Model file for the job. Use its own axes, mm. A direction names the side the tool comes from. Give positions to 0.01 mm unless a question says otherwise; leave off trailing zeros. Order: outer loops, then holes, each group sorted by start corner. A loop starts at its lowest first (then second) coordinate and runs counter-clockwise, first axis right, second up. Notation, with made-up numbers: M 45.5,-1.75 L 63.5,-1.75 A14 ccw 63.5,11.25 Z; hole C 46.25,-16.75 d2. An arc over 180 degrees is marked long. Return JSON: item names as keys, results as strings. Group by question number.
1. Slice it at A-A on y = 2. List the corners of the cut face in (x, z), then the cut area to 3 significant figures.
2. Two-plate mould, pull along X, no slides. Class faces 1 (the face through (-11.4, -20.43, -1.23)), 2 (the face through (-10, 23, 1)), 3 (the face through (11, -1.1, -2)), 4 (the face through (11.43, 24.4, -1.27)): released by +X, released by -X, zero draft, split by the parting line, or undercut.
3. Slice it at C-C on z = -1.6. List the corners of the cut face in (x, y), then the cut area to 3 significant figures.
4. Slice it at D-D on y = -16. List the corners of the cut face in (x, z), then the cut area to 3 significant figures.
5. Wall check: probe 1 along Y at (x, z) = (2.75, 0.35); probe 2 along X at (y, z) = (-15, 0.1); probe 3 along Z at (x, y) = (1.75, 18). Give the ranges that are in metal, low to high. Write a range as [from, to].
6. Slice it at B-B on x = 1.75. List the corners of the cut face in (y, z), then the cut area to 4 significant figures.
7. Pin check, flat tips, straight feed: pin 1 (0.6 mm diameter, centred on x = 11.5, z = -1.5, fed in from +Y); pin 2 (3 mm diameter, centred on y = 3, z = -1.5, fed in from +X); pin 3 (1.3 mm diameter, centred on y = 3.5, z = -2, fed in from -X); pin 4 (1 mm diameter, centred on x = 11, z = -2, fed in from -Y). Stop position of each tip, or through.
8. 3-axis set-ups, long thin cutter, end or side, ignore diameter. For faces 5 (the face through (11.4, -20.43, -1.27)), 6 (the face through (11, 2, -0.4)), 7 (the face through (-10, 2, -2)), 8 (the face through (0, 25, -1)), 9 (the face through (-10.699, 0.285, 0.247)): which of +Z, -Z, +X, -X, +Y, -Y reach the whole face in a straight line?
from build123d import *

# Parameters (mm, degrees)
BASE_DEPTH                = 3
CORNER_MARK_DEPTH         = 4.5
CORNER_MARK_DEPTH_BACK    = 4.5
CORNER_SKETCH_3_W         = 2
CORNER_SKETCH_3_H         = 0.5
CORNER_MARK_CUTOUT_DEPTH  = 0.75
CORNER_FIT_CUT_DEPTH      = 32.616432581
CORNER_FIT_CUT_DEPTH_BACK = 32.616432581
BORDER_START              = -3
BORDER_DEPTH              = 3.5
BODY_MIRROR_START         = -3
BODY_MIRROR_DEPTH         = 3
BODY_MIRROR_2_DEPTH       = 0.5
MAGNET_CUTOUT_SKETCH_W    = 2.6
MAGNET_CUTOUT_SKETCH_H    = 6.2
MAGNET_CUTOUT_DEPTH       = 2


with BuildPart() as part:
    # base_sketch → base (new body)
    with BuildSketch(Plane.XY):
        with BuildLine():
            ThreePointArc((-10, 0), (-10.707106781, 0.292893219), (-11, 1))
            Line((-11, 1), (-11, 23))
            ThreePointArc((-11, 23), (-10.707106781, 23.707106781), (-10, 24))
            Line((-10, 24), (0, 24))
            Line((0, 24), (0, 0))
            Line((0, 0), (-10, 0))
        make_face()
        with BuildLine():
            Line((0, -1), (-10, -1))
            ThreePointArc((-10, -1), (-10.707106781, -1.292893219), (-11, -2))
            Line((-11, -2), (-11, -19))
            ThreePointArc((-11, -19), (-10.707106781, -19.707106781), (-10, -20))
            Line((-10, -20), (0, -20))
            Line((0, -20), (0, -1))
        make_face()
        with BuildLine():
            Line((-10, 0), (0, 0))
            Line((0, 0), (0, -1))
            Line((0, -1), (-10, -1))
            ThreePointArc((-10, -1), (-10.707106781, -1.292893219), (-11, -2))
            Line((-11, -2), (-11, -19))
            ThreePointArc((-11, -19), (-10.707106781, -19.707106781), (-10, -20))
            Line((-10, -20), (0, -20))
            Line((0, -20), (0, -21))
            Line((0, -21), (-10, -21))
            ThreePointArc((-10, -21), (-11.414213562, -20.414213562), (-12, -19))
            Line((-12, -19), (-12, 23))
            ThreePointArc((-12, 23), (-11.414213562, 24.414213562), (-10, 25))
            Line((-10, 25), (0, 25))
            Line((0, 25), (0, 24))
            Line((0, 24), (-10, 24))
            ThreePointArc((-10, 24), (-10.707106781, 23.707106781), (-11, 23))
            Line((-11, 23), (-11, 1))
            ThreePointArc((-11, 1), (-10.707106781, 0.292893219), (-10, 0))
        make_face()
    extrude(amount=-BASE_DEPTH)

    # corner_sketch → corner_mark (add, two sides: drawn at the far end of the back side and taken through both)
    with BuildSketch(Plane(origin=(6.5, 6.5, 0), x_dir=(0.7071067811865477, -0.7071067811865475, 0), z_dir=(0.7071067811865475, 0.7071067811865477, 0)).offset(-CORNER_MARK_DEPTH_BACK)):
        with BuildLine():
            Line((-23.334523779, 0), (-25.334523779, 0))
            Line((-25.334523779, 0), (-25.334523779, -2))
            Line((-25.334523779, -2), (-23.748737342, -2))
            ThreePointArc((-23.748737342, -2), (-23.536817216, -1.97728699), (-23.334523779, -1.910179721))
            Line((-23.334523779, -1.910179721), (-23.334523779, 0))
        make_face()
        with BuildLine():
            Line((-21.334523779, 0), (-23.334523779, 0))
            Line((-23.334523779, 0), (-23.334523779, -1.910179721))
            ThreePointArc((-23.334523779, -1.910179721), (-23.178957136, -1.821797126), (-23.04163056, -1.707106781))
            Line((-23.04163056, -1.707106781), (-21.334523779, 0))
        make_face()
    extrude(amount=CORNER_MARK_DEPTH + CORNER_MARK_DEPTH_BACK)

    # corner_sketch<3> → corner_mark_cutout (cut, symmetric)
    with BuildSketch(Plane(origin=(6.5, 6.5, 0), x_dir=(0.7071067811865477, -0.7071067811865475, 0), z_dir=(0.7071067811865475, 0.7071067811865477, 0))):
        with BuildLine():
            Line((-21.334523779, 0), (-23.334523779, 0))
            Line((-23.334523779, 0), (-23.334523779, -1.910179721))
            ThreePointArc((-23.334523779, -1.910179721), (-23.178957136, -1.821797126), (-23.04163056, -1.707106781))
            Line((-23.04163056, -1.707106781), (-21.334523779, 0))
        make_face()
        with Locations((-22.334523779, 0.25)):
            Rectangle(CORNER_SKETCH_3_W, CORNER_SKETCH_3_H)
    extrude(amount=CORNER_MARK_CUTOUT_DEPTH, both=True, mode=Mode.SUBTRACT)

    # Эскиз3 → corner_fit_cut (cut, two sides: drawn at the far end of the back side and taken through both)
    with BuildSketch(Plane(origin=(0, 0, -3), x_dir=(-1, 0, 0), z_dir=(0, 0, -1)).offset(-CORNER_FIT_CUT_DEPTH_BACK)):
        with BuildLine():
            Line((10, 25), (4.949214827, 25))
            Line((4.949214827, 25), (4.949214827, 29.369186308))
            Line((4.949214827, 29.369186308), (15.830436382, 29.369186308))
            Line((15.830436382, 29.369186308), (15.830436382, 18.313069579))
            Line((15.830436382, 18.313069579), (12, 18.313069579))
            Line((12, 18.313069579), (12, 23))
            ThreePointArc((12, 23), (11.414213562, 24.414213562), (10, 25))
        make_face()
    extrude(amount=CORNER_FIT_CUT_DEPTH + CORNER_FIT_CUT_DEPTH_BACK, mode=Mode.SUBTRACT)

    # border: read off the stored shape, not the designer's step
    # border outline → border (add)
    with BuildSketch(Plane.XY.offset(BORDER_START)):
        Polygon((0, 24), (0, 25), (-5.878679656, 25), (-6.878679656, 24), align=None)
        with BuildLine():
            ThreePointArc((-10, 0), (-10.707106781, 0.292893219), (-11, 1))
            Line((-11, 1), (-11, 19.878679656))
            Line((-11, 19.878679656), (-12, 18.878679656))
            Line((-12, 18.878679656), (-12, -19))
            ThreePointArc((-12, -19), (-11.414213562, -20.414213562), (-10, -21))
            Line((-10, -21), (0, -21))
            Line((0, -21), (0, -20))
            Line((0, -20), (-10, -20))
            ThreePointArc((-10, -20), (-10.707106781, -19.707106781), (-11, -19))
            Line((-11, -19), (-11, -2))
            ThreePointArc((-11, -2), (-10.707106781, -1.292893219), (-10, -1))
            Line((-10, -1), (0, -1))
            Line((0, -1), (0, 0))
            Line((0, 0), (-10, 0))
        make_face()
    extrude(amount=BORDER_DEPTH)

    # body_mirror: read off the stored shape, not the designer's step
    # body_mirror outline → body_mirror (add)
    with BuildSketch(Plane.XY.offset(BODY_MIRROR_START)):
        with BuildLine():
            Line((0, -21), (10, -21))
            ThreePointArc((10, -21), (11.414213562, -20.414213562), (12, -19))
            Line((12, -19), (12, 23))
            ThreePointArc((12, 23), (11.414213562, 24.414213562), (10, 25))
            Line((10, 25), (0, 25))
            Line((0, 25), (0, -21))
        make_face()
    extrude(amount=BODY_MIRROR_DEPTH)

    # body_mirror 2 outline → body_mirror 2 (add)
    with BuildSketch(Plane.XY):
        with BuildLine():
            Line((0, -20), (0, -21))
            Line((0, -21), (10, -21))
            ThreePointArc((10, -21), (11.414213562, -20.414213562), (12, -19))
            Line((12, -19), (12, 23))
            ThreePointArc((12, 23), (11.414213562, 24.414213562), (10, 25))
            Line((10, 25), (0, 25))
            Line((0, 25), (0, 24))
            Line((0, 24), (10, 24))
            ThreePointArc((10, 24), (10.707106781, 23.707106781), (11, 23))
            Line((11, 23), (11, 1))
            ThreePointArc((11, 1), (10.707106781, 0.292893219), (10, 0))
            Line((10, 0), (0, 0))
            Line((0, 0), (0, -1))
            Line((0, -1), (10, -1))
            ThreePointArc((10, -1), (10.707106781, -1.292893219), (11, -2))
            Line((11, -2), (11, -19))
            ThreePointArc((11, -19), (10.707106781, -19.707106781), (10, -20))
            Line((10, -20), (0, -20))
        make_face()
    extrude(amount=BODY_MIRROR_2_DEPTH)

    # magnet_cutout_sketch → magnet_cutout (cut)
    with BuildSketch(Plane(origin=(12, 0, 0), x_dir=(0, 0, -1), z_dir=(1, 0, 0))):
        with Locations((1.7, 2)):
            Rectangle(MAGNET_CUTOUT_SKETCH_W, MAGNET_CUTOUT_SKETCH_H)
    magnet_cutout = extrude(amount=-MAGNET_CUTOUT_DEPTH, mode=Mode.SUBTRACT)

    # magnet_cutout_mirror: magnet_cutout across plane
    add(magnet_cutout.mirror(Plane(origin=(0, 0, 0), x_dir=(0, 0, 1), z_dir=(1, 0, 0))), mode=Mode.SUBTRACT)


solid = part.part
Result:
{
 "1": {"outline": "M -12,-0.4 L -10,-0.4 L -10,-3 L 10,-3 L 10,-0.4 L 12,-0.4 L 12,0.5 L 11,0.5 L 11,0 L -11,0 L -11,0.5 L -12,0.5 Z", "area": "62.6 mm2"},
 "2": {"face 1": "released by -X", "face 2": "undercut", "face 3": "zero draft", "face 4": "released by +X"},
 "3": {"outline": "M -12,-19 A2 ccw -10,-21 L 10,-21 A2 ccw 12,-19 L 12,-1.1 L 10,-1.1 L 10,5.1 L 12,5.1 L 12,23 A2 ccw 10,25 L -10,25 A2 ccw -12,23 L -12,5.1 L -10,5.1 L -10,-1.1 L -12,-1.1 Z", "area": "1,080 mm2"},
 "4": {"outline": "M -12,-3 L 12,-3 L 12,0.5 L 11,0.5 L 11,0 L -11,0 L -11,0.5 L -12,0.5 Z", "area": "73.0 mm2"},
 "5": {"probe 1": "y = [-21, -20], [-1, 0], [24, 25]", "probe 2": "x = [-12, -11], [11, 12]", "probe 3": "z = [-3, 0]"},
 "6": {"outline": "M -21,-3 L 25,-3 L 25,0.5 L 24,0.5 L 24,0 L 0,0 L 0,0.5 L -1,0.5 L -1,0 L -20,0 L -20,0.5 L -21,0.5 Z", "area": "139.5 mm2"},
 "7": {"pin 1": "stops at y = 24.6", "pin 2": "stops at x = 12", "pin 3": "stops at x = -10", "pin 4": "stops at y = -20.94"},
 "8": {"face 5": "+Z, -Z, +X, -Y", "face 6": "-Z, +X", "face 7": "-Z, -X", "face 8": "+Z, -Z, +X, -X, +Y", "face 9": "+Z"}
}
